Geometry check sheet. Reference: the model listing, model coordinates, mm. A direction names the side the tool comes from. Coordinates: 2 decimals unless noted, no trailing zeros. Loops run counter-clockwise (first coordinate to the right, second up) from the corner with the lowest first, then second, coordinate; pieces in that order, holes last.
from build123d import *

# Parameters (mm, degrees)
F0_R     = 12.2
F1_DEPTH = 7


with BuildPart() as f1:
    # F0 (on Top) → F1 (new body)
    with BuildSketch(Plane.XY):
        with BuildLine():
            ThreePointArc((-10.461899, 16.917701), (-7.259172, 14.314915), (-3.443284, 12.74299))
            ThreePointArc((-3.443284, 12.74299), (-11.431535, 6.6), (-12.757395, -3.389524))
            ThreePointArc((-12.757395, -3.389524), (-16.111427, -0.823731), (-20.071696, 0.642248))
            ThreePointArc((-20.071696, 0.642248), (-21.411446, 0.855021), (-22.765386, 0.938982))
            ThreePointArc((-22.765386, 0.938982), (-35.073825, -20.679014), (-10.224124, -19.526737))
            ThreePointArc((-10.224124, -19.526737), (-9.783892, -18.538255), (-9.420209, -17.51912))
            ThreePointArc((-9.420209, -17.51912), (-8.767494, -13.444085), (-9.314111, -9.353466))
            ThreePointArc((-9.314111, -9.353466), (0, -13.2), (9.314111, -9.353466))
            ThreePointArc((9.314111, -9.353466), (8.769085, -13.541039), (9.479645, -17.703722))
            ThreePointArc((9.479645, -17.703722), (9.965253, -18.970367), (10.569511, -20.184894))
            ThreePointArc((10.569511, -20.184894), (35.445464, -20.035316), (22.022712, 0.909018))
            ThreePointArc((22.022712, 0.909018), (20.946546, 0.796028), (19.882108, 0.60142))
            ThreePointArc((19.882108, 0.60142), (16.026666, -0.870831), (12.757395, -3.389524))
            ThreePointArc((12.757395, -3.389524), (11.431535, 6.6), (3.443284, 12.74299))
            ThreePointArc((3.443284, 12.74299), (7.342341, 14.36477), (10.592051, 17.061474))
            ThreePointArc((10.592051, 17.061474), (11.446193, 18.115346), (12.195875, 19.245912))
            ThreePointArc((12.195875, 19.245912), (-0.371639, 40.71433), (-11.798589, 18.617719))
            ThreePointArc((-11.798589, 18.617719), (-11.162654, 17.742227), (-10.461899, 16.917701))
        make_face()
        with Locations((-22.966296, -13.259597)):
            Circle(F0_R, mode=Mode.SUBTRACT)
        with Locations((22.966296, -13.259597)):
            Circle(F0_R, mode=Mode.SUBTRACT)
        Circle(F0_R, mode=Mode.SUBTRACT)
        with Locations((0, 26.519194)):
            Circle(F0_R, mode=Mode.SUBTRACT)
        with BuildLine():
            ThreePointArc((-20.071696, 0.642248), (-13.280016, 7.606885), (-10.461899, 16.917701))
            ThreePointArc((-10.461899, 16.917701), (-11.162654, 17.742227), (-11.798589, 18.617719))
            ThreePointArc((-11.798589, 18.617719), (-15.442187, 8.637052), (-22.765386, 0.938982))
            ThreePointArc((-22.765386, 0.938982), (-21.411446, 0.855021), (-20.071696, 0.642248))
        make_face()
        with BuildLine():
            ThreePointArc((22.022712, 0.909018), (15.201, 9.054801), (12.195875, 19.245912))
            ThreePointArc((12.195875, 19.245912), (11.446193, 18.115346), (10.592051, 17.061474))
            ThreePointArc((10.592051, 17.061474), (13.227764, 7.697389), (19.882108, 0.60142))
            ThreePointArc((19.882108, 0.60142), (20.946546, 0.796028), (22.022712, 0.909018))
        make_face()
        with BuildLine():
            ThreePointArc((-9.420209, -17.51912), (-9.783892, -18.538255), (-10.224124, -19.526737))
            ThreePointArc((-10.224124, -19.526737), (0.241187, -17.691853), (10.569511, -20.184894))
            ThreePointArc((10.569511, -20.184894), (9.965253, -18.970367), (9.479645, -17.703722))
            ThreePointArc((9.479645, -17.703722), (0.052253, -15.304274), (-9.420209, -17.51912))
        make_face()
    extrude(amount=F1_DEPTH)


solid = f1.part
1) Section check C-C on x = 0. Record the cut outline in (y, z).
Data:
outline: (-17.69, 0) - (-15.3, 0) - (-15.3, 7) - (-17.69, 7) - close; (-13.2, 0) - (-12.2, 0) - (-12.2, 7) - (-13.2, 7) - close; (12.2, 0) - (14.32, 0) - (14.32, 7) - (12.2, 7) - close; (38.72, 0) - (40.72, 0) - (40.72, 7) - (38.72, 7) - close
2) Depth check by flat-ended pin: pin 1 (4 mm diameter, centred on x = 17.5, z = 4, fed in from +Y); pin 2 (1.5 mm diameter, centred on y = -10, z = 5, fed in from +X); pin 3 (1.5 mm diameter, centred on x = 1, y = 11, fed in from -Z). Enter the tip coordinate at first touch or a pass-through.
Data:
pin 1: stops at y = 8.51
pin 2: stops at x = 36.94
pin 3: passes through
3) Mould release check, pull along Y, two halves, no side actions. Record for faces 1 (the flat face through (-6, -11, 0)), 2 (the cylindrical face through (-35.3, -20.3, 3.5)), 3 (the cylindrical face through (15.272, 8.923, 3.451)): +Y half, -Y half, draft (parallel to the pull), parting line (faces both ways), or undercut.
Data:
face 1: draft
face 2: parting line
face 3: undercut
4) Section check D-D on z = 5. Record the cut outline in (x, y).
Data:
outline: (-22.77, 0.94) arc R14.2 ccw (long way) to (-10.22, -19.53) arc R26.07 cw to (10.57, -20.18) arc R14.2 ccw (long way) to (22.02, 0.91) arc R26.07 cw to (12.2, 19.25) arc R14.2 ccw (long way) to (-11.8, 18.62) arc R26.07 cw to start; hole circle Ø24.4 at (-22.97, -13.26); hole (-20.07, 0.64) arc R14.2 cw to (-12.76, -3.39) arc R13.2 cw to (-3.44, 12.74) arc R14.2 cw to (-10.46, 16.92) arc R20.51 cw to start; hole circle Ø24.4 at (0, 0); hole circle Ø24.4 at (0, 26.52); hole (-9.42, -17.52) arc R20.51 cw to (9.48, -17.7) arc R14.2 cw to (9.31, -9.35) arc R13.2 cw to (-9.31, -9.35) arc R14.2 cw to start; hole (3.44, 12.74) arc R13.2 cw to (12.76, -3.39) arc R14.2 cw to (19.88, 0.6) arc R20.51 cw to (10.59, 17.06) arc R14.2 cw to start; hole circle Ø24.4 at (22.97, -13.26)
5) Access from +Z, -Z, +X, -X, +Y, -Y to the whole of each face (thin tool, end or side, straight path). Record for faces 4 (the cylindrical face through (-31.958, -5.014, 3.451)), 5 (the cylindrical face through (-15.364, 8.765, 3.451)).
Data:
face 4: +Z, -Z
face 5: +Z, -Z, -X
6) Section check B-B on x = 31.5. Record the cut outline in (y, z).
Data:
outline: (-24.61, 0) - (-21.98, 0) - (-21.98, 7) - (-24.61, 7) - close; (-4.54, 0) - (-1.91, 0) - (-1.91, 7) - (-4.54, 7) - close
7) Material ranges on probe 1 along Y at (x, z) = (0, 2); probe 2 along X at (y, z) = (-13.5, 4.25); probe 3 along X at (y, z) = (-3, 3.5), recorded low to high.
Data:
probe 1: y = -17.69 to -15.3, -13.2 to -12.2, 12.2 to 14.32, 38.72 to 40.72
probe 2: x = -37.16 to -35.16, -10.77 to -8.77, 8.77 to 10.77, 35.16 to 37.16
probe 3: x = -32.78 to -29.57, -16.36 to -13.15, -12.85 to -11.83, 11.83 to 12.85, 13.15 to 16.36, 29.57 to 32.78
8) Section check A-A on y = 35. Record the cut outline in (x, z), and give its area (3 significant figures).
Data:
outline: (-11.39, 0) - (-8.77, 0) - (-8.77, 7) - (-11.39, 7) - close; (8.77, 0) - (11.39, 0) - (11.39, 7) - (8.77, 7) - close
area: 36.7 mm2
